```python
from build123d import *

# Parameters (mm, degrees)
SKETCH_3_W          = 8
SKETCH_3_H          = 16.823898374
CUT_EXTRUDE_1_DEPTH = 10
SKETCH_5_OUTSIDE_W  = 23.858
SKETCH_5_OUTSIDE_H  = 27.858
SKETCH_5_OUTSIDE_R  = 7.77784742
CUT_EXTRUDE_2_DEPTH = 10
SKETCH_6_R          = 3
EXTRUDE_1_DEPTH     = 6


with BuildPart() as part:
    # 草图2 → 旋转1 (revolve)
    with BuildSketch(Plane(origin=(0, 0, 0), x_dir=(0, 0, -1), z_dir=(1, 0, 0))):
        Polygon((0, 0), (0, 4), (15, 4), (15, 9), (21, 9), (21, 4), (32, 4), (32, 0), align=None)
    revolve(axis=Axis((0, 0, 0), (0, 0, -1)))

    # 草图3 → 切除-拉伸1 (cut)
    with BuildSketch(Plane.XY.offset(-15)):
        with Locations((-11, -0.026043186)):
            Rectangle(SKETCH_3_W, SKETCH_3_H)
        with Locations((11, -0.026043186)):
            Rectangle(SKETCH_3_W, SKETCH_3_H)
    extrude(amount=-CUT_EXTRUDE_1_DEPTH, mode=Mode.SUBTRACT)

    # 草图5 outside → 切除-拉伸2 (cut)
    with BuildSketch(Plane(origin=(0, 0, -21), x_dir=(-1, 0, 0), z_dir=(0, 0, -1))):
        Rectangle(SKETCH_5_OUTSIDE_W, SKETCH_5_OUTSIDE_H)
        Circle(SKETCH_5_OUTSIDE_R, mode=Mode.SUBTRACT)
    extrude(amount=-CUT_EXTRUDE_2_DEPTH, mode=Mode.SUBTRACT)

    # 草图6 → 凸台-拉伸1 (add)
    with BuildSketch(Plane(origin=(0, 0, -32), x_dir=(-1, 0, 0), z_dir=(0, 0, -1))):
        Circle(SKETCH_6_R)
    extrude(amount=EXTRUDE_1_DEPTH)


solid = part.part
```
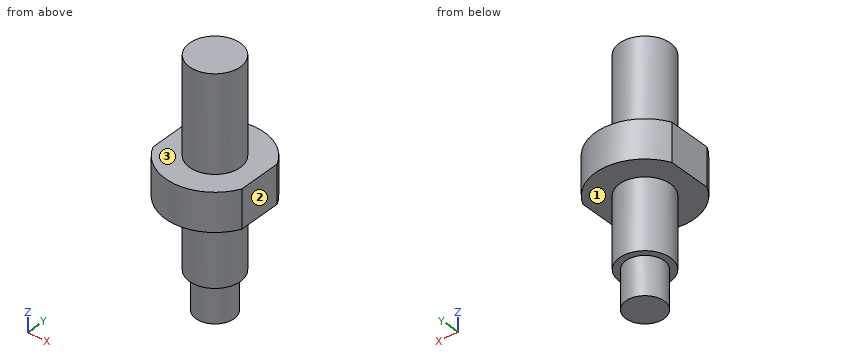
Build history of the part. All positions in model axes, mm. Face numbers are marked on the shaded views. A direction names the side the tool comes from. Round coordinates to 2 decimals unless told otherwise and drop trailing zeros. Write each loop counter-clockwise with the first axis right and the second up, starting at its lowest first coordinate (ties: lowest second). Pieces come first, ordered by that corner, then holes. Notation, with made-up numbers: (-28.75, -18) - (-21.75, -18) arc R16 ccw to (-21.75, 6) - close; hole circle Ø3 at (30, 40). An arc over 180 degrees is marked (long way). Answer as CSV lines item,"result".
Q1. Cut at C-C (z = -16). Write the cut outline in (x, y), and give its area (3 significant figures).
Report:
outline,"(-7, -3.39) arc R7.78 ccw to (7, -3.39) - (7, 3.39) arc R7.78 ccw to (-7, 3.39) - close"
area,"183 mm^2"
Q2. Drop flat-ended pins along their axis: pin 1 (1 mm diameter, centred on x = -2.5, z = -33.5, fed in from -Y); pin 2 (6 mm diameter, centred on x = -4, z = -11.5, fed in from +Y); pin 3 (1 mm diameter, centred on x = 4.5, y = -3.5, fed in from -Z). Give the stop position or say it passes through.
Report:
pin 1,"stops at y = -2.24"
pin 2,"stops at y = 3.87"
pin 3,"stops at z = -21"
Q3. Drill centre lines: probe 1 along Z at (x, y) = (-1.5, 3); probe 2 along Z at (x, y) = (-0.25, -4.5); probe 3 along Y at (x, z) = (2.5, -6.5). Where is each one in solid material? Low to high. Write a range as [from, to].
Report:
probe 1,"z = [-32, 0]"
probe 2,"z = [-21, -15]"
probe 3,"y = [-3.12, 3.12]"
Q4. Cut at B-B (y = 0). Write the cut outline in (x, z), and give its area (3 significant figures).
Report:
outline,"(-7, -21) - (-4, -21) - (-4, -32) - (-3, -32) - (-3, -38) - (3, -38) - (3, -32) - (4, -32) - (4, -21) - (7, -21) - (7, -15) - (4, -15) - (4, 0) - (-4, 0) - (-4, -15) - (-7, -15) - close"
area,"328 mm^2"
Q5. Cut at A-A (x = 0). Write the cut outline in (y, z), and give its area (3 significant figures).
Report:
outline,"(-7.78, -21) - (-4, -21) - (-4, -32) - (-3, -32) - (-3, -38) - (3, -38) - (3, -32) - (4, -32) - (4, -21) - (7.78, -21) - (7.78, -15) - (4, -15) - (4, 0) - (-4, 0) - (-4, -15) - (-7.78, -15) - close"
area,"337 mm^2"
Q6. Tool access for the marked faces 1, 2 and 3: list every direction of +Z, -Z, +X, -X, +Y, -Y with a clear straight run to the whole face (end or side of a thin tool).
Report:
face 1,"-Z"
face 2,"+Z, -Z, +X, +Y, -Y"
face 3,"+Z"
Q7. Cut at D-D (y = -6.25). Write the cut outline in (x, z).
Report:
outline,"(-4.63, -21) - (4.63, -21) - (4.63, -15) - (-4.63, -15) - close"
